The model under review builds one solid part; all positions refer to its coordinate system, in mm. Face numbers are marked on the shaded views. A direction names the side the tool comes from. Give positions to 0.01 mm unless a question says otherwise; leave off trailing zeros. Write each loop counter-clockwise with the first axis right and the second up, starting at its lowest first coordinate (ties: lowest second). Pieces come first, ordered by that corner, then holes. Notation, with made-up numbers: (-9.75, -21) - (7.25, -21) arc R20 ccw to (7.25, -5) - close; hole circle Ø8 at (71.25, 20). An arc over 180 degrees is marked (long way). One line per question, with ' | ' between items. Start each with the question number.
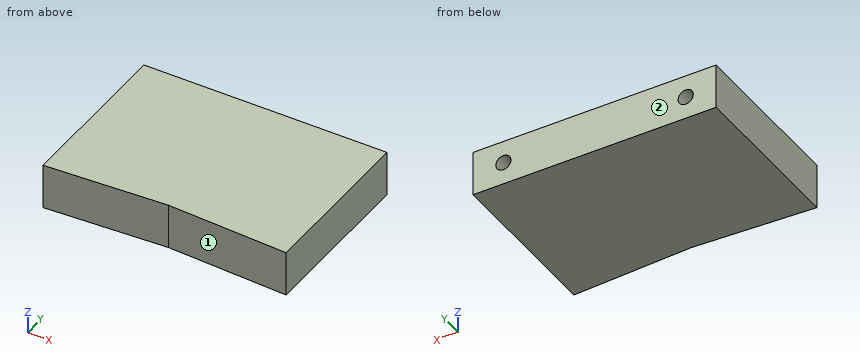
```python
from build123d import *

# Parameters (mm, degrees)
SKETCH1_W             = 80
SKETCH1_H             = 14.88
BOSS_EXTRUDE1_DEPTH   = 55.2
CUT_EXTRUDE1_DEPTH    = 70.774310459
M6_TAPPED_HOLE1_D     = 5
M6_TAPPED_HOLE1_DEPTH = 15
M6_TAPPED_HOLE1_TIP   = 1.502151548


with BuildPart() as part:
    # Sketch1 → Boss-Extrude1 (new body)
    with BuildSketch(Plane(origin=(0, 0, 0), x_dir=(1, 0, 0), z_dir=(0, 1, 0))):
        Rectangle(SKETCH1_W, SKETCH1_H)
    extrude(amount=-BOSS_EXTRUDE1_DEPTH)

    # Sketch3 → Cut-Extrude1 (cut, through all)
    with BuildSketch(Plane(origin=(0, 0, -7.44), x_dir=(-1, 0, 0), z_dir=(0, 0, -1))):
        Polygon((40, -55.2), (0, -53.103688829), (-40, -55.2), align=None)
    extrude(amount=-CUT_EXTRUDE1_DEPTH, mode=Mode.SUBTRACT)

    # M6 Tapped Hole1
    with Locations(Plane(origin=(0, 0, 0), x_dir=(1, 0, 0), z_dir=(0, 1, 0))):
        with Locations((-30, 0), (30, 0)):
            Hole(M6_TAPPED_HOLE1_D / 2, depth=M6_TAPPED_HOLE1_DEPTH)
            with Locations((0, 0, -(M6_TAPPED_HOLE1_DEPTH + M6_TAPPED_HOLE1_TIP / 2))):  # 118° drill point
                Cone(0, M6_TAPPED_HOLE1_D / 2, M6_TAPPED_HOLE1_TIP, mode=Mode.SUBTRACT)


solid = part.part
```
Item 1: Take a section at A-A (z = -3.5). Give the boundary of the cut face in (x, y).
Item 2: Clearance check with flat-ended pins moving along their axes: P1, Ø6.5, axis at x = -30, z = 0, coming from the -Y side; P2, Ø3, axis at x = 30, z = 0, coming from the +Y side. State where each tip first meets the part, or that it passes through.
Item 3: For probe 1 along Z at (x, y) = (-30, -11); probe 2 along Z at (x, y) = (28.5, -4); probe 3 along Y at (x, z) = (34, -3.5), list the stretches that pass through material, from the lowest coordinate up.
Item 4: Take a section at D-D (x = 17). Give the boundary of the cut face in (y, z).
Item 5: Machinability: for the marked faces 1 and 2, which of the approach directions +Z, -Z, +X, -X, +Y, -Y give a long, thin tool a straight path to every point of the face, cutting with its end or side? Answer none if there is none.
Item 6: Take a section at C-C (x = -21). Give the boundary of the cut face in (y, z), plus the area to 3 significant figures.
Item 7: Take a section at B-B (y = -8). Give the boundary of the cut face in (x, z), plus the area to 3 significant figures.
Check sheet entries:
1) outline: (-40, -55.2) - (0, -53.1) - (40, -55.2) - (40, 0) - (-40, 0) - close
2) P1: stops at y = -54.85 | P2: stops at y = -15.6
3) probe 1: z = -7.44 to -2.5, 2.5 to 7.44 | probe 2: z = -7.44 to -2, 2 to 7.44 | probe 3: y = -54.89 to 0
4) outline: (-53.99, -7.44) - (0, -7.44) - (0, 7.44) - (-53.99, 7.44) - close
5) face 1: +Z, -Z, -Y | face 2: +Z, -Z, +X, -X, +Y
6) outline: (-54.2, -7.44) - (0, -7.44) - (0, 7.44) - (-54.2, 7.44) - close | area: 807 mm^2
7) outline: (-40, -7.44) - (40, -7.44) - (40, 7.44) - (-40, 7.44) - close; hole circle Ø5 at (-30, 0); hole circle Ø5 at (30, 0) | area: 1,150 mm^2
